Verification items for the finished model (mm, model axes). A direction names the side the tool comes from. Round coordinates to 2 decimals unless told otherwise and drop trailing zeros. Order: outer loops, then holes, each group sorted by start corner. A loop starts at its lowest first (then second) coordinate and runs counter-clockwise, first axis right, second up.
```python
from build123d import *

# Parameters (mm, degrees)
F0_R      = 3
F0_R_2    = 2.499
F1_DEPTH  = 0.5
F0_R_3    = 1.999
F2_DEPTH  = 7.95
F3_R      = 2.75
F3_R_2    = 2.499
F3_R_3    = 1.999
F4_DEPTH  = 1
F6_DEPTH  = 3
F7_R      = 2.75
F7_R_2    = 2.499
F8_DEPTH  = 1
F10_DEPTH = 3
F11_DEPTH = 0.05
F12_DEPTH = 0.05
F13_DEPTH = 0.45
F14_DEPTH = 0.45


with BuildPart() as f1:
    # F0 (on Front) → F1 (new body, symmetric)
    with BuildSketch(Plane.XZ):
        Circle(F0_R)
        Circle(F0_R_2, mode=Mode.SUBTRACT)
    extrude(amount=F1_DEPTH, both=True)

    # F0 (on Front) → F2 (join, symmetric)
    with BuildSketch(Plane.XZ):
        Circle(F0_R_2)
        Circle(F0_R_3, mode=Mode.SUBTRACT)
    extrude(amount=F2_DEPTH, both=True)

    # F3 (on face) → F4 (join)
    with BuildSketch(Plane.XZ.offset(7.95)):
        Circle(F3_R)
        Circle(F3_R_2, mode=Mode.SUBTRACT)
        Circle(F3_R_2)
        Circle(F3_R_3, mode=Mode.SUBTRACT)
    extrude(amount=-F4_DEPTH)

    # F5 (on face) → F6 (cut)
    with BuildSketch(Plane.XZ.offset(7.95)):
        with BuildLine():
            Line((1.983305574, -0.25), (2.7386127875, -0.25))
            ThreePointArc((2.7386127875, -0.25), (2.75, 0), (2.7386127875, 0.25))
            Line((2.7386127875, 0.25), (1.983305574, 0.25))
            ThreePointArc((1.983305574, 0.25), (1.999, 0), (1.983305574, -0.25))
        make_face()
        with BuildLine():
            ThreePointArc((-1.983305574, -0.25), (-1.999, 0), (-1.983305574, 0.25))
            Line((-1.983305574, 0.25), (-2.7386127875, 0.25))
            ThreePointArc((-2.7386127875, 0.25), (-2.75, 0), (-2.7386127875, -0.25))
            Line((-2.7386127875, -0.25), (-1.983305574, -0.25))
        make_face()
    extrude(amount=-F6_DEPTH, mode=Mode.SUBTRACT)

    # F7 (on face) → F8 (join)
    with BuildSketch(Plane(origin=(0, 7.95, 0), x_dir=(-1, 0, 0), z_dir=(0, 1, 0))):
        Circle(F7_R)
        Circle(F7_R_2, mode=Mode.SUBTRACT)
    extrude(amount=-F8_DEPTH)

    # F9 (on face) → F10 (cut)
    with BuildSketch(Plane(origin=(0, 7.95, 0), x_dir=(-1, 0, 0), z_dir=(0, 1, 0))):
        with BuildLine():
            ThreePointArc((2.7386127875, -0.25), (2.75, 0), (2.7386127875, 0.25))
            Line((2.7386127875, 0.25), (1.983305574, 0.25))
            ThreePointArc((1.983305574, 0.25), (1.999, 0), (1.983305574, -0.25))
            Line((1.983305574, -0.25), (2.7386127875, -0.25))
        make_face()
        with BuildLine():
            Line((-1.983305574, 0.25), (-2.7386127875, 0.25))
            ThreePointArc((-2.7386127875, 0.25), (-2.75, 0), (-2.7386127875, -0.25))
            Line((-2.7386127875, -0.25), (-1.983305574, -0.25))
            ThreePointArc((-1.983305574, -0.25), (-1.999, 0), (-1.983305574, 0.25))
        make_face()
    extrude(amount=-F10_DEPTH, mode=Mode.SUBTRACT)

    # F11 (cut): faces of the model
    f11_faces = [f1.faces().sort_by_distance(p)[0] for p in [
        (-2.3609591808, 7.95, 0.3102079729),
        (2.2442931831, 4.95, 0),
        (0, 7.95, -2.6897920271),
        (-2.2442931831, 4.95, 0),
    ]]
    extrude(f11_faces, amount=-F11_DEPTH, mode=Mode.SUBTRACT)

    # F12 (cut): faces of the model
    f12_faces = [f1.faces().sort_by_distance(p)[0] for p in [
        (0, -7.95, 2.0592079729),
        (-2.2442931831, -4.95, 0),
        (2.3609591808, -7.95, -0.3102079729),
        (2.2442931831, -4.95, 0),
    ]]
    extrude(f12_faces, amount=-F12_DEPTH, mode=Mode.SUBTRACT)

    # F13 (cut): faces of the model
    f13_faces = [f1.faces().sort_by_distance(p)[0] for p in [
        (-2.6125381702, 6.95, 0.3102079729),
        (0, 6.95, -2.6897920271),
    ]]
    extrude(f13_faces, amount=-F13_DEPTH, mode=Mode.SUBTRACT)

    # F14 (cut): faces of the model
    f14_faces = [f1.faces().sort_by_distance(p)[0] for p in [
        (2.6125381702, -6.95, 0.3102079729),
        (0, -6.95, -2.6897920271),
    ]]
    extrude(f14_faces, amount=-F14_DEPTH, mode=Mode.SUBTRACT)


solid = f1.part
```
1) Sectioned sample at D-D on y = -1. Record the cut outline in (x, z), then the cut area to 3 significant figures.
2) Sectioned sample at C-C on x = -1.3. Record the cut outline in (y, z).
3) Tool access check on faces 5 (the cylindrical face through (-0.06, 7.65, 2.75)), 6 (the cylindrical face through (-0.06, -7.65, -2.75)), 7 (the flat face through (-2, -0.5, 2)). Record the directions out of +Z, -Z, +X, -X, +Y, -Y that give a thin tool (end or side, any length) a straight path to the whole face; none if there is none.
4) Scan lines: probe 1 along Z at (x, y) = (0, 4.5); probe 2 along Z at (x, y) = (1.35, 5.25). Record each from-to range of solid material in increasing order.
5) Sectioned sample at B-B on z = 0. Record the cut outline in (x, y).
6) Go/stop test with flat-tipped pins: pin 1 Ø1 at (x, y) = (1, 0) entering from -Z; pin 2 Ø1 at (x, y) = (0, 2.5) entering from -Z; pin 3 Ø0.8 at (x, y) = (-2.5, 6.5) entering from +Z; pin 4 Ø3 at (x, z) = (0, 0) entering from -Y. Record where each tip stops, or that it passes through.
7) Draft check along Y on faces 1 (the cylindrical face through (0.06, -7.65, 2.75)), 2 (the flat face through (-2, 0.5, 2)), 3 (the flat face through (1, -7.9, -2)), 4 (the flat face through (-1, 7.9, -2)). Enter one of: released by +Y, released by -Y, zero draft, split by the parting line, or undercut.
Returned:
1. outline: circle Ø5 at (0, 0); hole circle Ø4 at (0, 0)
1. area: 7.07 mm2
2. outline: (-7.9, -2.42) - (-7.4, -2.42) - (-7.4, -2.13) - (-0.5, -2.13) - (-0.5, -2.7) - (0.5, -2.7) - (0.5, -2.13) - (7.4, -2.13) - (7.4, -2.42) - (7.9, -2.42) - (7.9, -1.52) - (-7.9, -1.52) - close; (-7.9, 1.52) - (7.9, 1.52) - (7.9, 2.42) - (7.4, 2.42) - (7.4, 2.13) - (0.5, 2.13) - (0.5, 2.7) - (-0.5, 2.7) - (-0.5, 2.13) - (-7.4, 2.13) - (-7.4, 2.42) - (-7.9, 2.42) - close
3. face 5: +Z, +Y
3. face 6: -Z, -Y
3. face 7: none
4. probe 1: z = -2.5 to -2, 2 to 2.5
4. probe 2: z = -2.1 to -1.47, 1.47 to 2.1
5. outline: (-3, -0.5) - (-2.5, -0.5) - (-2.5, -4.9) - (-2, -4.9) - (-2, 4.9) - (-2.5, 4.9) - (-2.5, 0.5) - (-3, 0.5) - close; (2, -4.9) - (2.5, -4.9) - (2.5, -0.5) - (3, -0.5) - (3, 0.5) - (2.5, 0.5) - (2.5, 4.9) - (2, 4.9) - close
6. pin 1: stops at z = -2.96
6. pin 2: stops at z = -2.5
6. pin 3: stops at z = 1.35
6. pin 4: passes through
7. face 1: zero draft
7. face 2: undercut
7. face 3: released by -Y
7. face 4: released by +Y
